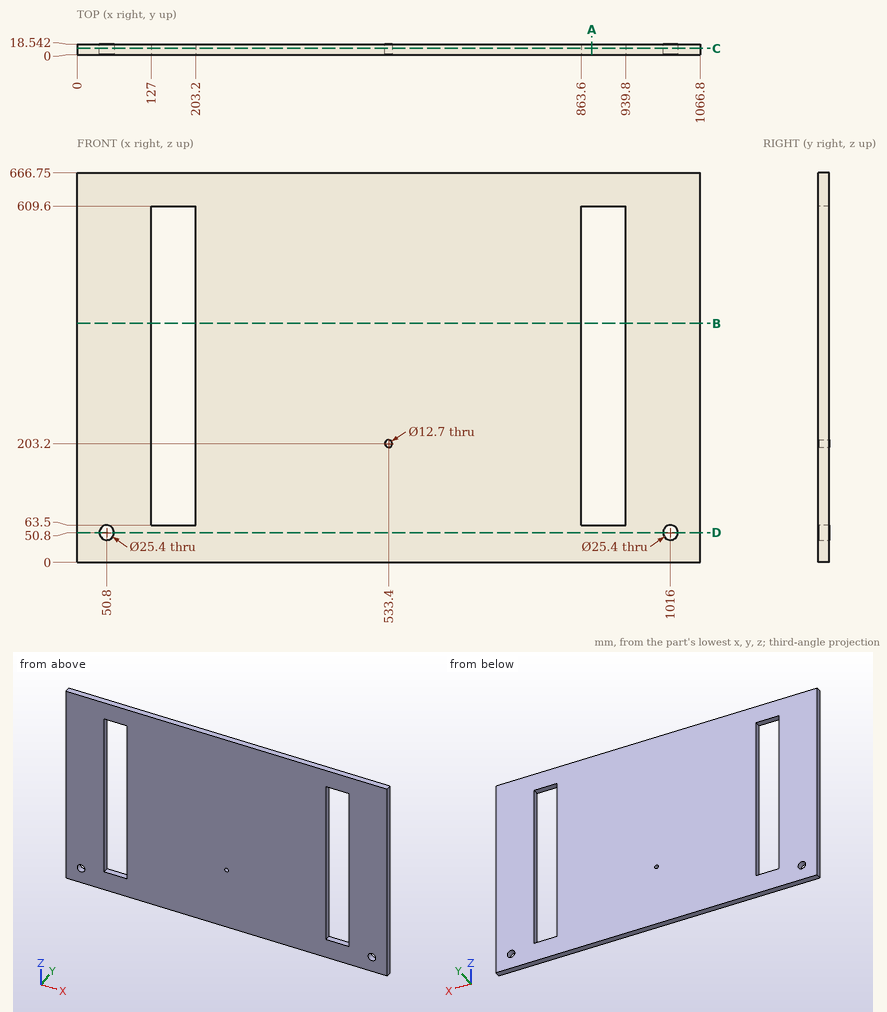
Part print with two shaded views. Sizes in mm from the minimum x, y, z corner. Coordinates: 2 decimals unless noted, no trailing zeros. Write each loop counter-clockwise with the first axis right and the second up, starting at its lowest first coordinate (ties: lowest second). Pieces come first, ordered by that corner, then holes. Notation, with made-up numbers: (31, 28) - (64, 28) arc R25 cw to (64, 50) - close; hole circle Ø8 at (24, 24.25). An arc over 180 degrees is marked (long way). Use a Markdown table: item, result. Add a question column.
Item 1: Band-saw the part on C-C, the plane y = 11. Write the cut outline in (x, z).
Item 2: Band-saw the part on A-A, the plane x = 881.5. Write the cut outline in (y, z).
Item 3: Band-saw the part on B-B, the plane z = 409. Write the cut outline in (x, y), and give its area (3 significant figures).
Item 4: Drill centre lines: line 1 along X through (y, z) = (16.25, 300); line 2 along Z through (x, y) = (153, 6); line 3 along Z through (x, y) = (533.4, 13.25). Where is each one in solid material? Low to high.
Item 5: Band-saw the part on D-D, the plane z = 50.8. Write the cut outline in (x, y), and give its area (3 significant figures).
A:
| question | item | result |
|---|---|---|
| 1 | outline | (0, 0) - (1066.8, 0) - (1066.8, 666.75) - (0, 666.75) - close; hole circle Ø25.4 at (50.8, 50.8); hole (127, 63.5) - (203.2, 63.5) - (203.2, 609.6) - (127, 609.6) - close; hole circle Ø12.7 at (533.4, 203.2); hole (863.6, 63.5) - (939.8, 63.5) - (939.8, 609.6) - (863.6, 609.6) - close; hole circle Ø25.4 at (1016, 50.8) |
| 2 | outline | (0, 0) - (18.54, 0) - (18.54, 63.5) - (0, 63.5) - close; (0, 609.6) - (18.54, 609.6) - (18.54, 666.75) - (0, 666.75) - close |
| 3 | outline | (0, 0) - (127, 0) - (127, 18.54) - (0, 18.54) - close; (203.2, 0) - (863.6, 0) - (863.6, 18.54) - (203.2, 18.54) - close; (939.8, 0) - (1066.8, 0) - (1066.8, 18.54) - (939.8, 18.54) - close |
| 3 | area | 17,000 mm² |
| 4 | line 1 | x = 0 to 127, 203.2 to 863.6, 939.8 to 1066.8 |
| 4 | line 2 | z = 0 to 63.5, 609.6 to 666.75 |
| 4 | line 3 | z = 0 to 196.85, 209.55 to 666.75 |
| 5 | outline | (0, 0) - (38.1, 0) - (38.1, 18.54) - (0, 18.54) - close; (63.5, 0) - (1003.3, 0) - (1003.3, 18.54) - (63.5, 18.54) - close; (1028.7, 0) - (1066.8, 0) - (1066.8, 18.54) - (1028.7, 18.54) - close |
| 5 | area | 18,800 mm² |
